from build123d import *

# Parameters (mm, degrees)
F0_R     = 18.5
F0_R_2   = 17.5
F1_DEPTH = 30
F0_R_3   = 16.5
F2_DEPTH = 1.5
F3_SIZE  = 0.5


with BuildPart() as f1:
    # F0 (on Top) → F1 (new body)
    with BuildSketch(Plane.XY):
        Circle(F0_R)
        Circle(F0_R_2, mode=Mode.SUBTRACT)
    extrude(amount=F1_DEPTH)

    # F0 (on Top) → F2 (join)
    with BuildSketch(Plane.XY):
        Circle(F0_R_2)
        Circle(F0_R_3, mode=Mode.SUBTRACT)
    extrude(amount=F2_DEPTH)

    # F3
    f3_edges = [f1.edges().sort_by_distance(p)[0] for p in [
        (-18.5, 0, 0),
        (-16.5, 0, 0),
    ]]
    chamfer(f3_edges, length=F3_SIZE)


solid = f1.part
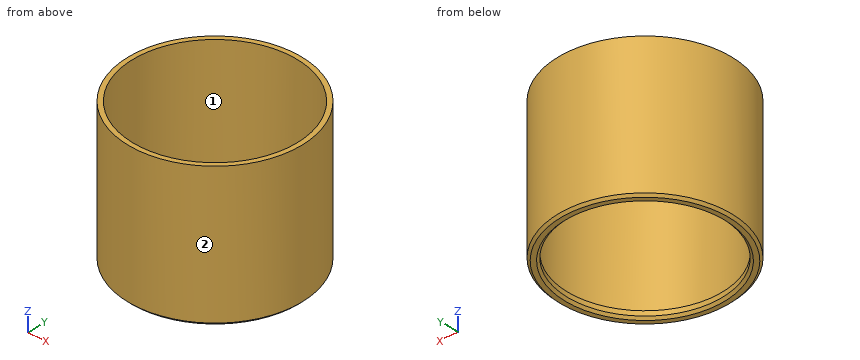
Check sheet for the modelled part. Datum: model origin and axes. Units: mm. Face numbers are marked on the shaded views. Round coordinates to 2 decimals unless told otherwise and drop trailing zeros. Order: outer loops, then holes, each group sorted by start corner. A loop starts at its lowest first (then second) coordinate and runs counter-clockwise, first axis right, second up.
(1) Scan lines: probe 1 along Y at (x, z) = (0, 1.1); probe 2 along Y at (x, z) = (0, 20.25); probe 3 along X at (y, z) = (14, 15.5). Record each from-to range of solid material in increasing order.
(2) Go/stop test with flat-tipped pins: P1, Ø1.5, axis at y = -4.5, z = 12.5, coming from the +X side; P2, Ø3, axis at x = 5.5, z = 5, coming from the +Y side; P3, Ø3, axis at y = 14, z = 17, coming from the -X side. Record where each tip stops, or that it passes through.
(3) Cross-section at A-A, the plane x = 0. Enter the section's corners in (y, z), and give its area (3 significant figures).
(4) Draft check along Y on the marked faces 1 and 2. Enter one of: pulls with the +Y half, pulls with the -Y half, needs draft (parallel to the pull), parting line crosses it, or undercut.
(5) Cross-section at C-C, the plane z = 9. Enter the section's corners in (x, y), and give its area (3 significant figures).
Check sheet entries:
1. probe 1: y = -18.5 to -16.5, 16.5 to 18.5
1. probe 2: y = -18.5 to -17.5, 17.5 to 18.5
1. probe 3: x = -12.09 to -10.5, 10.5 to 12.09
2. P1: stops at x = 18.12
2. P2: stops at y = 18.06
2. P3: stops at x = -13.64
3. outline: (-18.5, 0.5) - (-18, 0) - (-17, 0) - (-16.5, 0.5) - (-16.5, 1.5) - (-17.5, 1.5) - (-17.5, 30) - (-18.5, 30) - close; (16.5, 0.5) - (17, 0) - (18, 0) - (18.5, 0.5) - (18.5, 30) - (17.5, 30) - (17.5, 1.5) - (16.5, 1.5) - close
3. area: 62.5 mm2
4. face 1: undercut
4. face 2: parting line crosses it
5. outline: circle Ø37 at (0, 0); hole circle Ø35 at (0, 0)
5. area: 113 mm2
